CAD build for the part. Positions are in the model's coordinates, mm. A direction names the side the tool comes from. Give positions to 0.01 mm unless a question says otherwise; leave off trailing zeros. Write each loop counter-clockwise with the first axis right and the second up, starting at its lowest first coordinate (ties: lowest second). Pieces come first, ordered by that corner, then holes. Notation, with made-up numbers: (66, -26.5) - (122, -26.5) arc R26 cw to (122, -3.5) - close; hole circle Ø4 at (36, 88). An arc over 180 degrees is marked (long way). Put each result on its own line as item: value. Start each with the question number.
1. Wall check: line 1 (X direction, y = 52.5, z = 84.5); line 2 (Y direction, x = 24, z = 240); line 3 (Z direction, x = 231, y = 22). Give the ranges that are in metal, low to high.
2. Cut at A-A on z = 11.5. List the corners of the cut face in (x, y).
3. Drop flat-ended pins along their axis: pin 1 (10 mm diameter, centred on x = -159, y = 72.5, fed in from -Z); pin 2 (3 mm diameter, centred on y = 54.5, z = 226.5, fed in from -X); pin 3 (22 mm diameter, centred on y = 39, z = -94, fed in from +X); pin 4 (6 mm diameter, centred on x = 41.5, z = -93, fed in from -Y). Give the stop position or say it passes through.
4. Cut at C-C on z = 127. List the corners of the cut face in (x, y).
5. Cut at B-B on z = -38.5. List the corners of the cut face in (x, y), and give its area (3 significant figures).
6. Tool access for faces 4 (the cylindrical face through (153.11, 14.85, 91.28)), 5 (the flat face through (-167, 48, -89.759)), 6 (the flat face through (239.808, 48, 197)), 7 (the cylindrical face through (161.98, 84.14, 73.48)), 8 (the flat face through (238, 47, 113.241)): list every direction of +Z, -Z, +X, -X, +Y, -Y with a clear straight run to the whole face (end or side of a thin tool).
7. Mould opens along X. For faces 1 (the flat face through (-235.192, 47, -76)), 2 (the flat face through (87, 78, -96)), 3 (the flat face through (152, 47, 216.241)) say: +X half, -X half, draft (parallel to the pull), parting line (faces both ways), or undercut.
from build123d import *

# Parameters (mm, degrees)
BOSS_EXTRUDE1_DEPTH      = 96
BOSS_EXTRUDE2_START      = -96
SKETCH2_R                = 164
SKETCH2_R_2              = 112.5
BOSS_EXTRUDE2_DEPTH      = 96
SKETCH3_R                = 10
CUT_EXTRUDE2_DEPTH       = 22
CIRPATTERN1_COUNT        = 8
SKETCH4_R                = 8
CUT_EXTRUDE3_DEPTH       = 26
CIRPATTERN2_COUNT        = 8
FILLET1_R                = 10
CUT_EXTRUDE4_DEPTH       = 391.958919102
CUT_EXTRUDE4_DEPTH_BACK  = 391.958919102
CUT_EXTRUDE5_DEPTH       = 391.958919102
CUT_EXTRUDE5_DEPTH_BACK  = 2
SKETCH6_R                = 155
SKETCH7_R                = 164
CUT_EXTRUDE6_DEPTH       = 4
CUT_EXTRUDE7_DEPTH       = 391.958919102
CUT_EXTRUDE7_DEPTH_BACK  = 391.958919102
SKETCH8_W                = 24
SKETCH8_H                = 60
CUT_EXTRUDE8_DEPTH       = 470.945214053
CUT_EXTRUDE8_DEPTH_BACK  = 470.945214053
SKETCH9_W                = 24
SKETCH9_H                = 60
CUT_EXTRUDE9_DEPTH       = 530.537885533
CUT_EXTRUDE9_DEPTH_BACK  = 530.537885533
SKETCH10_R               = 11
CUT_EXTRUDE10_DEPTH      = 428.606716751
CUT_EXTRUDE10_DEPTH_BACK = 428.606716751
SKETCH11_R               = 13


with BuildPart() as part:
    # Sketch1 → Boss-Extrude1 (new body)
    with BuildSketch(Plane(origin=(0, 0, 0), x_dir=(1, 0, 0), z_dir=(0, 1, 0))):
        with BuildLine():
            Line((-96.191532686, 101.75916217), (-235.191532686, 101.75916217))
            Line((-235.191532686, 101.75916217), (-235.191532686, 48.75916217))
            Line((-235.191532686, 48.75916217), (-175.191532686, 48.75916217))
            Line((-175.191532686, 48.75916217), (-175.191532686, 45.75916217))
            Line((-175.191532686, 45.75916217), (-172.191532686, 45.75916217))
            ThreePointArc((-172.191532686, 45.75916217), (-150.978329251, 36.972365606), (-142.191532686, 15.75916217))
            Line((-142.191532686, 15.75916217), (-142.191532686, -83.24083783))
            ThreePointArc((-142.191532686, -83.24083783), (21.808467314, 80.75916217), (185.808467314, -83.24083783))
            ThreePointArc((185.808467314, -83.24083783), (167.8089992, -157.939195837), (117.761580864, -216.24083783))
            Line((117.761580864, -216.24083783), (183.808467314, -216.24083783))
            ThreePointArc((183.808467314, -216.24083783), (194.415069031, -220.634236112), (198.808467314, -231.24083783))
            Line((198.808467314, -231.24083783), (201.808467314, -234.24083783))
            Line((201.808467314, -234.24083783), (201.808467314, -283.24083783))
            Line((201.808467314, -283.24083783), (251.808467314, -283.24083783))
            Line((251.808467314, -283.24083783), (251.808467314, -113.24083783))
            Line((251.808467314, -113.24083783), (231.808467314, -113.24083783))
            Line((231.808467314, -113.24083783), (231.808467314, -53.24083783))
            Line((231.808467314, -53.24083783), (251.808467314, -53.24083783))
            Line((251.808467314, -53.24083783), (251.808467314, 45.75916217))
            Line((251.808467314, 45.75916217), (251.808467314, 101.75916217))
            Line((251.808467314, 101.75916217), (-36.191532686, 101.75916217))
            Line((-36.191532686, 101.75916217), (-36.191532686, 81.75916217))
            Line((-36.191532686, 81.75916217), (-96.191532686, 81.75916217))
            Line((-96.191532686, 81.75916217), (-96.191532686, 101.75916217))
        make_face()
    extrude(amount=BOSS_EXTRUDE1_DEPTH)

    # Sketch2 → Boss-Extrude2 (add)
    with BuildSketch(Plane(origin=(0, 96, 0), x_dir=(1, 0, 0), z_dir=(0, 1, 0)).offset(BOSS_EXTRUDE2_START)):
        with Locations((21.808467314, -83.24083783)):
            Circle(SKETCH2_R)
        with Locations(Location((21.808467314, -83.24083783, 0), (0, 0, 270))):
            Circle(SKETCH2_R_2, mode=Mode.SUBTRACT)
    extrude(amount=BOSS_EXTRUDE2_DEPTH)

    # Sketch3 → Cut-Extrude2 (cut)
    with BuildSketch(Plane(origin=(0, 96, 0), x_dir=(1, 0, 0), z_dir=(0, 1, 0))):
        with Locations(Location((21.808467314, 54.75916217, 0), (0, 0, 270))):
            Circle(SKETCH3_R)
    cut_extrude2 = extrude(amount=-CUT_EXTRUDE2_DEPTH, mode=Mode.SUBTRACT)

    # CirPattern1: Cut-Extrude2 ×8 about axis
    cirpattern1_axis = Axis((21.808467314, 0, 83.24083783), (0, 1, 0))
    for i in range(1, CIRPATTERN1_COUNT):
        add(cut_extrude2.rotate(cirpattern1_axis, i * 360 / CIRPATTERN1_COUNT), mode=Mode.SUBTRACT)

    # Sketch4 → Cut-Extrude3 (cut)
    with BuildSketch(Plane(origin=(0, 0, 0), x_dir=(-1, 0, 0), z_dir=(0, -1, 0))):
        with Locations(Location((-20.864768315, -218.23753939, 0), (0, 0, 90))):
            Circle(SKETCH4_R)
    cut_extrude3 = extrude(amount=-CUT_EXTRUDE3_DEPTH, mode=Mode.SUBTRACT)

    # CirPattern2: Cut-Extrude3 ×8 about axis
    cirpattern2_axis = Axis((21.808467314, 0, 83.24083783), (0, 1, 0))
    for i in range(1, CIRPATTERN2_COUNT):
        add(cut_extrude3.rotate(cirpattern2_axis, i * 360 / CIRPATTERN2_COUNT), mode=Mode.SUBTRACT)

    # Fillet1
    fillet1_edges = [part.edges().sort_by_distance(p)[0] for p in [
        (117.761580864, 48, 216.24083783),
    ]]
    fillet(fillet1_edges, radius=FILLET1_R)

    # Sketch5 → Cut-Extrude4 (cut, two sides: drawn at the far end of the back side and taken through both)
    with BuildSketch(Plane(origin=(0, 96, 0), x_dir=(1, 0, 0), z_dir=(0, 1, 0)).offset(-CUT_EXTRUDE4_DEPTH_BACK)):
        Polygon((251.808467314, 101.75916217), (201.808467314, 101.75916217), (251.808467314, 51.75916217), align=None)
    extrude(amount=CUT_EXTRUDE4_DEPTH + CUT_EXTRUDE4_DEPTH_BACK, mode=Mode.SUBTRACT)

    # Sketch6 → Cut-Extrude5 (cut, two sides: drawn at the far end of the back side and taken through both)
    with BuildSketch(Plane(origin=(0, 96, 0), x_dir=(1, 0, 0), z_dir=(0, 1, 0)).offset(-CUT_EXTRUDE5_DEPTH_BACK)):
        with Locations(Location((21.808467314, -83.24083783, 0), (0, 0, 90))):
            Circle(SKETCH6_R)
    extrude(amount=CUT_EXTRUDE5_DEPTH + CUT_EXTRUDE5_DEPTH_BACK, mode=Mode.SUBTRACT)

    # Sketch7 → Cut-Extrude6 (cut)
    with BuildSketch(Plane.XZ):
        with Locations((21.808467314, 83.24083783)):
            Circle(SKETCH7_R)
    extrude(amount=-CUT_EXTRUDE6_DEPTH, mode=Mode.SUBTRACT)

    # Sketch8 → Cut-Extrude7 (cut, two sides: drawn at the far end of the back side and taken through both)
    with BuildSketch(Plane(origin=(0, 0, 0), x_dir=(0, 0, -1), z_dir=(1, 0, 0)).offset(-CUT_EXTRUDE7_DEPTH_BACK)):
        with Locations((101.75916217, 48)):
            Rectangle(SKETCH8_W, SKETCH8_H)
    extrude(amount=CUT_EXTRUDE7_DEPTH + CUT_EXTRUDE7_DEPTH_BACK, mode=Mode.SUBTRACT)

    # Sketch9 → Cut-Extrude8 (cut, two sides: drawn at the far end of the back side and taken through both)
    with BuildSketch(Plane.XY.offset(283.24083783).offset(-CUT_EXTRUDE8_DEPTH_BACK)):
        with Locations((251.808467314, 48)):
            Rectangle(SKETCH9_W, SKETCH9_H)
    extrude(amount=CUT_EXTRUDE8_DEPTH + CUT_EXTRUDE8_DEPTH_BACK, mode=Mode.SUBTRACT)

    # Sketch10 → Cut-Extrude9 (cut, two sides: drawn at the far end of the back side and taken through both)
    with BuildSketch(Plane.ZY.offset(-201.808467314).offset(-CUT_EXTRUDE9_DEPTH_BACK)):
        with BuildLine():
            Line((266.100753095, 33), (266.100753095, 22))
            Line((266.100753095, 22), (277.100753095, 22))
            ThreePointArc((277.100753095, 22), (273.878927688, 29.778174593), (266.100753095, 33))
        make_face()
        with BuildLine():
            Line((277.100753095, 22), (266.100753095, 22))
            Line((266.100753095, 22), (266.100753095, 33))
            ThreePointArc((266.100753095, 33), (258.322578502, 14.221825407), (277.100753095, 22))
        make_face()
        with Locations(Location((266.100753095, 74, 0), (0, 0, 21.323686263))):
            Circle(SKETCH10_R)
    extrude(amount=CUT_EXTRUDE9_DEPTH + CUT_EXTRUDE9_DEPTH_BACK, mode=Mode.SUBTRACT)

    # Sketch11 → Cut-Extrude10 (cut, two sides: drawn at the far end of the back side and taken through both)
    with BuildSketch(Plane.XY.offset(-48.75916217).offset(-CUT_EXTRUDE10_DEPTH_BACK)):
        with Locations(Location((-210.191532686, 72, 0), (0, 0, 27.48642625))):
            Circle(SKETCH11_R)
        with Locations(Location((-210.191532686, 24, 0), (0, 0, 332.51357375))):
            Circle(SKETCH11_R)
    extrude(amount=CUT_EXTRUDE10_DEPTH + CUT_EXTRUDE10_DEPTH_BACK, mode=Mode.SUBTRACT)


solid = part.part
Report:
1. line 1: x = -142.19 to -90.68, 134.3 to 231.81
1. line 2: y = 4 to 96
1. line 3: z = -72.57 to 255.1, 277.1 to 283.24
2. outline: (-142.19, 0) - (-125.67, 0) - (-125.67, 4) - (-64.85, 4) - (-64.85, 94) - (-115.59, 94) - (-115.59, 96) - (-142.19, 96) - close; (108.47, 4) - (169.28, 4) - (169.28, 0) - (251.81, 0) - (251.81, 18) - (239.81, 18) - (239.81, 78) - (251.81, 78) - (251.81, 96) - (159.21, 96) - (159.21, 94) - (108.47, 94) - close
3. pin 1: stops at z = -89.76
3. pin 2: stops at x = -60.66
3. pin 3: stops at x = 220.57
3. pin 4: stops at y = 0
4. outline: (-136.25, 4) - (-81.83, 4) - (-81.83, 94) - (-126.89, 94) - (-126.89, 96) - (-136.25, 96) - close; (125.45, 4) - (179.86, 4) - (179.86, 0) - (251.81, 0) - (251.81, 18) - (239.81, 18) - (239.81, 78) - (251.81, 78) - (251.81, 96) - (170.5, 96) - (170.5, 94) - (125.45, 94) - close
5. outline: (-152.62, 0) - (-88.08, 0) - (-88.08, 4) - (131.7, 4) - (131.7, 0) - (251.81, 0) - (251.81, 18) - (239.81, 18) - (239.81, 78) - (251.81, 78) - (251.81, 96) - (117.75, 96) - (117.75, 94) - (-74.13, 94) - (-74.13, 96) - (-152.62, 96) - close
5. area: 36,800 mm²
6. face 4: -Y
6. face 5: -Z, +X, -X
6. face 6: +Z, -Z, +X
6. face 7: +Y
6. face 8: +X, +Y, -Y
7. face 1: -X half
7. face 2: draft
7. face 3: undercut
